Build history of the part. All positions in model axes, mm. A direction names the side the tool comes from. Give positions to 0.01 mm unless a question says otherwise; leave off trailing zeros. Order: outer loops, then holes, each group sorted by start corner. A loop starts at its lowest first (then second) coordinate and runs counter-clockwise, first axis right, second up. Notation, with made-up numbers: (46, 7.25) -> (78, 7.25) arc R32 ccw to (78, 44.25) -> close; hole circle Ø9 at (-18.5, 56). An arc over 180 degrees is marked (long way). One line per item, written item: value. Start each with the question number.
(1) Saw through at C-C on y = 28. Give the cut face in (x, z), plus the area to 3 significant figures.
(2) Pin check, flat tips, straight feed: pin 1 (5 mm diameter, centred on x = 23.5, z = 19, fed in from +Y); pin 2 (14 mm diameter, centred on x = 0.12, y = 0, fed in from +Z); pin 3 (3 mm diameter, centred on y = -17, z = 33.5, fed in from +X). Stop position of each tip, or through.
(3) Probe line 1 (Z direction, x = -29.5, y = -10.5); line 2 (Y direction, x = -25, z = 31.25); line 3 (X direction, y = 30.5, z = 22.75). List the from-to ranges inside material, lowest first.
(4) Saw through at B-B on z = 21.25. Give the cut face in (x, y), plus the area to 3 significant figures.
(5) Which spindle directions (+Z, -Z, +X, -X, +Y, -Y) get a long thin tool onto all of the face, cutting with end or side? Do faces 5 (the cylindrical face through (0.38, 26.82, 25.37)), 6 (the flat face through (-3.884, 14, 14)), 7 (the flat face through (4.116, 14, 14)). Say none if no direction does.
(6) Saw through at A-A on y = -9. Give the cut face in (x, z), plus the area to 3 significant figures.
(7) Two-plate mould, pull along X, no slides. Class faces 1 (the cylindrical face through (-26.67, -13.63, 25.37)), 2 (the cylindrical face through (-8.271, 5.012, 14.52)), 3 (the cylindrical face through (-33.67, -19.064, 14.52)), 4 (the cylindrical face through (0.498, 38.794, 14.52)): +X half, -X half, draft (parallel to the pull), parting line (faces both ways), or undercut.
(8) Saw through at D-D on x = -18. Give the cut face in (y, z).
```python
from build123d import *

# Parameters (mm, degrees)
BOSS_EXTRUDE2_DEPTH = 10
SKETCH3_R           = 50
BOSS_EXTRUDE3_DEPTH = 10
SKETCH4_R           = 10
BOSS_EXTRUDE4_DEPTH = 90
CUT_EXTRUDE1_START  = -30
SKETCH5_R           = 10
CUT_EXTRUDE1_DEPTH  = 30
SKETCH6_R           = 13
CUT_EXTRUDE2_DEPTH  = 10
SKETCH7_R           = 10
BOSS_EXTRUDE5_DEPTH = 30
SKETCH9_R           = 10
BOSS_EXTRUDE6_DEPTH = 10
SKETCH10_R          = 10
BOSS_EXTRUDE7_DEPTH = 10
SKETCH11_R          = 10
BOSS_EXTRUDE8_DEPTH = 10
SKETCH12_R          = 50
BOSS_EXTRUDE9_DEPTH = 10
SKETCH13_R          = 30
CUT_EXTRUDE3_DEPTH  = 10
SCALE1_SCALE        = 0.2


with BuildPart() as part:
    # Sketch1 → Boss-Extrude2 (new body)
    with BuildSketch(Plane.XY):
        Polygon((20, 144), (-20, 144), (-20, 11.547005384), (-134.707658145, -54.679491924), (-114.707658145, -89.320508076), (0, -23.094010768), (114.707658145, -89.320508076), (134.707658145, -54.679491924), (20, 11.547005384), align=None)
    extrude(amount=BOSS_EXTRUDE2_DEPTH)

    # Sketch3 → Boss-Extrude3 (add)
    with BuildSketch(Plane.XY.offset(10)):
        with Locations((-124.707658145, -72)):
            Circle(SKETCH3_R)
        with Locations((0, 144)):
            Circle(SKETCH3_R)
        with Locations((124.707658145, -72)):
            Circle(SKETCH3_R)
    extrude(amount=-BOSS_EXTRUDE3_DEPTH)

    # Sketch4 → Boss-Extrude4 (add)
    with BuildSketch(Plane.XY.offset(10)):
        with Locations(Location((0, 144, 0), (0, 0, 180))):
            Circle(SKETCH4_R)
        with Locations(Location((124.707658145, -72, 0), (0, 0, 180))):
            Circle(SKETCH4_R)
        with Locations(Location((-124.707658145, -72, 0), (0, 0, 180))):
            Circle(SKETCH4_R)
    extrude(amount=BOSS_EXTRUDE4_DEPTH)

    # Sketch5 → Cut-Extrude1 (cut)
    with BuildSketch(Plane.XY.offset(100).offset(CUT_EXTRUDE1_START)):
        with Locations(Location((0, 144, 0), (0, 0, 180))):
            Circle(SKETCH5_R)
    extrude(amount=CUT_EXTRUDE1_DEPTH, mode=Mode.SUBTRACT)

    # Sketch6 → Cut-Extrude2 (cut)
    with BuildSketch(Plane.XY.offset(10)):
        Circle(SKETCH6_R)
    extrude(amount=-CUT_EXTRUDE2_DEPTH, mode=Mode.SUBTRACT)

    # Sketch7 → Boss-Extrude5 (add)
    with BuildSketch(Plane.XY.offset(70)):
        with Locations(Location((0, 144, 0), (0, 0, 180))):
            Circle(SKETCH7_R)
    extrude(amount=BOSS_EXTRUDE5_DEPTH)

    # Sketch9 → Boss-Extrude6 (add)
    with BuildSketch(Plane.XY.offset(100)):
        with Locations(Location((0, 144, 0), (0, 0, 180))):
            Circle(SKETCH9_R)
    extrude(amount=BOSS_EXTRUDE6_DEPTH)

    # Sketch10 → Boss-Extrude7 (add)
    with BuildSketch(Plane.XY.offset(100)):
        with Locations(Location((-124.707658145, -72, 0), (0, 0, 180))):
            Circle(SKETCH10_R)
    extrude(amount=BOSS_EXTRUDE7_DEPTH)

    # Sketch11 → Boss-Extrude8 (add)
    with BuildSketch(Plane.XY.offset(100)):
        with Locations(Location((124.707658145, -72, 0), (0, 0, 180))):
            Circle(SKETCH11_R)
    extrude(amount=BOSS_EXTRUDE8_DEPTH)

    # Sketch12 → Boss-Extrude9 (add)
    with BuildSketch(Plane.XY.offset(10)):
        with Locations((1.330805308, 0)):
            Circle(SKETCH12_R)
    extrude(amount=-BOSS_EXTRUDE9_DEPTH)

    # Sketch13 → Cut-Extrude3 (cut)
    with BuildSketch(Plane.XY.offset(10)):
        Circle(SKETCH13_R)
    extrude(amount=-CUT_EXTRUDE3_DEPTH, mode=Mode.SUBTRACT)


with BuildPart() as part_1:
    # Scale1: scaled about (0.145453699, 0.001217976, 16.882898765)
    add(part.part.scale(SCALE1_SCALE).moved(Location((0.116362959, 0.000974381, 13.506319012))))


solid = part_1.part
```
Results below:
1. outline: (-9.85, 13.51) -> (10.08, 13.51) -> (10.08, 15.51) -> (1.95, 15.51) -> (1.95, 35.51) -> (-1.72, 35.51) -> (-1.72, 15.51) -> (-9.85, 15.51) -> close
1. area: 113 mm²
2. pin 1: stops at y = -12.4
2. pin 2: stops at z = 15.51
2. pin 3: stops at x = 26.73
3. line 1: z = 13.51 to 15.51
3. line 2: y = -16.39 to -12.41
3. line 3: x = -0.94 to 1.17
4. outline: circle Ø4 at (-24.83, -14.4); circle Ø4 at (0.12, 28.8); circle Ø4 at (25.06, -14.4)
4. area: 37.7 mm²
5. face 5: +Z
5. face 6: +Z, -Z, -X
5. face 7: +Z, -Z, +X
6. outline: (-33.24, 13.51) -> (-7.47, 13.51) -> (-7.47, 15.51) -> (-33.24, 15.51) -> close; (-3.97, 13.51) -> (4.74, 13.51) -> (4.74, 15.51) -> (-3.97, 15.51) -> close; (7.71, 13.51) -> (33.48, 13.51) -> (33.48, 15.51) -> (7.71, 15.51) -> close
6. area: 121 mm²
7. face 1: undercut
7. face 2: -X half
7. face 3: undercut
7. face 4: parting line
8. outline: (-21.71, 13.51) -> (-5.84, 13.51) -> (-5.84, 15.51) -> (-21.71, 15.51) -> close
